For this review, take the finished solid that the model builds, in its own axes (mm). Face numbers are marked on the shaded views. Coordinates: 2 decimals unless noted, no trailing zeros. Order: outer loops, then holes, each group sorted by start corner. A loop starts at its lowest first (then second) coordinate and runs counter-clockwise, first axis right, second up. Notation, with made-up numbers: (80.25, 77) - (87.25, 77) arc R7 cw to (87.25, 90) - close; hole circle Ø7 at (-21, 33.25). An arc over 180 degrees is marked (long way). One line per item, written item: value. Start each with the question number.
(1) Mouldability with a two-part tool opening along X and no side actions: class the marked faces 1, 2 and 3 as released by +X, released by -X, zero draft, split by the parting line, or undercut.
(2) Consider section A-A on z = 105.5. Write out the cut boundary in (x, y).
(3) Consider section B-B on y = 0. Write out the cut boundary in (x, z).
(4) Clearance check with flat-ended pins moving along their axes: pin 1 (3 mm diameter, centred on y = -2, z = 14.5, fed in from -X); pin 2 (4 mm diameter, centred on x = 7.5, z = 106.5, fed in from +Y) (3 decimals); pin 3 (8.5 mm diameter, centred on x = 2.5, y = 1.5, fed in from -Z); pin 4 (4 mm diameter, centred on x = 8.5, y = 1.5, fed in from -Z). State where each tip first meets the part, or that it passes through.
(5) To check wall thickness, follow line 1 along X through (y, z) = (0, 60); line 2 along Z through (x, y) = (5.75, -1); line 3 along X through (y, z) = (4.5, 105.5). State the ranges of each line that lie inside material, in increasing order.
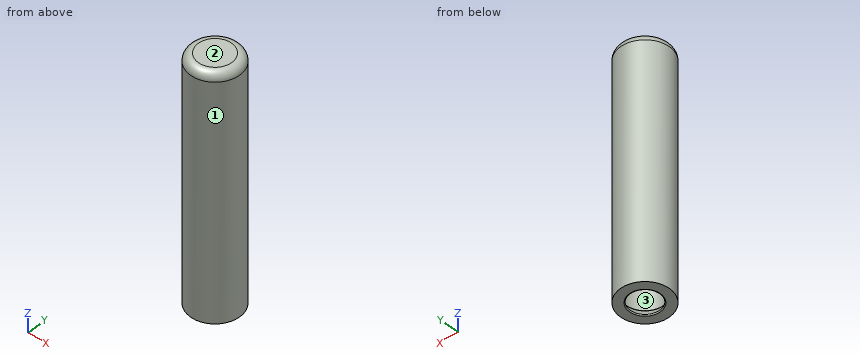
Autodesk Inventor part; units mm, degrees
ref_plane "YZ Plane" through (0, 0, 0) normal (1, 0, 0) x (0, 1, 0)
ref_plane "XZ Plane" through (0, 0, 0) normal (0, 1, 0) x (-1, 0, 0)
ref_plane "XY Plane" through (0, 0, 0) normal (0, 0, 1) x (1, 0, 0)
sketch "Sketch4" plane through (0, 0, 0) normal (1, 0, 0) x (0, 1, 0)
  line L0 (-12.5, 0) -> (12.5, 0)
  line L1 (-12.5, 0) -> (-9.5, 0)
  line L2 (-9.5, 4.0551) -> (-9.5, 119)
  line L3 (0, 120) -> (0, 123)
  line L4 (0, 123) -> (-8.5, 123)
  arc A0 (-8.5, 123) -> (-12.5, 119) centre (-8.5, 119) ccw
  line L5 (-12.5, 119) -> (-12.5, 0)
  line L6 (-8.5, 120) -> (0, 120)
  arc A1 (-8.5, 120) -> (-9.5, 119) centre (-8.5, 119) ccw
  line L7 (-9.5, 0) -> (-7.9135, 0)
  line L8 (-7.5671, 0.6) -> (-9.4464, 3.8551)
  line L9 (-7.2207, 0) -> (-1.4448, 0) construction
  arc A2 (-9.5, 4.0551) -> (-9.4464, 3.8551) centre (-9.1, 4.0551) ccw
  arc A3 (-7.9135, 0) -> (-7.5671, 0.6) centre (-7.9135, 0.4) ccw
  point P0 (0, 0)
  point P1 (-9.5, 120)
  point P2 (-6.5, 0)
  point P3 (-9.5, 3.9479)
  dimension "d7" = 120
  dimension "d8" = 3
  dimension "d9" = 4
  dimension "d10" = 1
  dimension "d11" = 3
  dimension "d14" = 120
  dimension "d15" = 0.4
revolve "Revolution1" add sketch "Sketch4" angle 360 about axis through (0, 0, 120) along (0, 0, 1)
properties part number "Diffueser"
Geometry check:
1. face 1: split by the parting line
1. face 2: zero draft
1. face 3: undercut
2. outline: circle Ø25 at (0, 0); hole circle Ø19 at (0, 0)
3. outline: (-12.5, 0) - (-7.91, 0) arc R0.4 ccw to (-7.57, 0.6) - (-9.45, 3.86) arc R0.4 cw to (-9.5, 4.06) - (-9.5, 119) arc R1 cw to (-8.5, 120) - (8.5, 120) arc R1 cw to (9.5, 119) - (9.5, 4.06) arc R0.4 cw to (9.45, 3.86) - (7.57, 0.6) arc R0.4 ccw to (7.91, 0) - (12.5, 0) - (12.5, 119) arc R4 ccw to (8.5, 123) - (-8.5, 123) arc R4 ccw to (-12.5, 119) - close
4. pin 1: stops at x = -12.49
4. pin 2: stops at y = 11.225
4. pin 3: stops at z = 120
4. pin 4: stops at z = 0
5. line 1: x = -12.5 to -9.5, 9.5 to 12.5
5. line 2: z = 120 to 123
5. line 3: x = -11.66 to -8.37, 8.37 to 11.66
